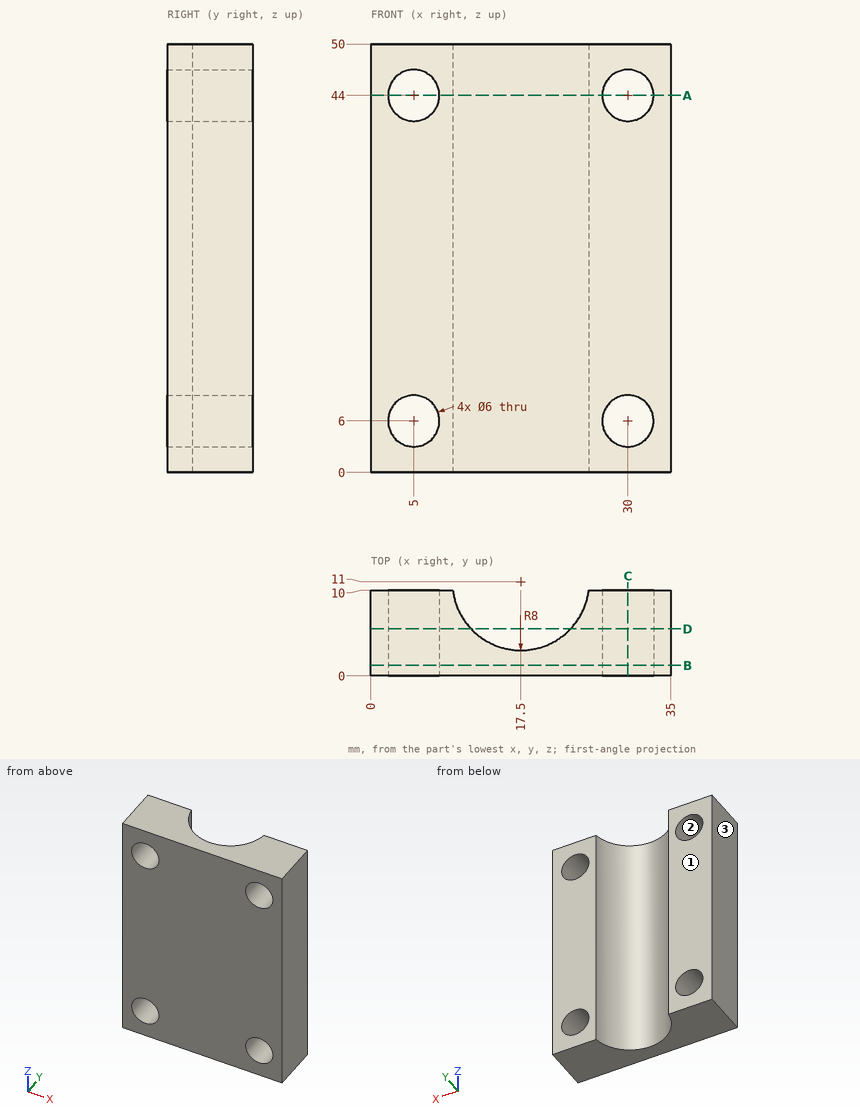
The drawing under review shows one solid part. Ordinate dimensions are in mm from its lowest x, y, z. Coordinates: 2 decimals unless noted, no trailing zeros. Order: outer loops, then holes, each group sorted by start corner. A loop starts at its lowest first (then second) coordinate and runs counter-clockwise, first axis right, second up. Notation, with made-up numbers: (-20.5, 56.5) -> (7.5, 56.5) arc R25 cw to (7.5, 93.5) -> close; hole circle Ø10 at (-37.75, 6.5). An arc over 180 degrees is marked (long way). Answer in a Markdown table with one row per item. Add a question column.
Item 1: We need section D-D on y = 5.5. Write out the cut boundary in (x, z).
Item 2: We need section C-C on x = 30. Write out the cut boundary in (y, z).
Item 3: We need section B-B on y = 1.25. Write out the cut boundary in (x, z), plus the area to 3 significant figures.
Item 4: To check wall thickness, follow probe 1 along X at (y, z) = (2.5, 44); probe 2 along Z at (x, y) = (31, 3.75); probe 3 along X at (y, z) = (8.25, 6). State the ranges of each line that lie inside material, in increasing order.
Item 5: Clearance check with a flat-ended pin moving along its axis: pin 1 (4 mm diameter, centred on x = 7, z = 21.5, fed in from -Y). State where the tip first meets the part, or that it passes through.
Item 6: Mouldability with a two-part tool opening along X and no side actions: class the marked faces 1, 2 and 3 as +X half, -X half, draft (parallel to the pull), parting line (faces both ways), or undercut.
Item 7: We need section A-A on z = 44. Write out the cut boundary in (x, y).
Final values:
| question | item | result |
|---|---|---|
| 1 | outline | (0, 0) -> (11.69, 0) -> (11.69, 50) -> (0, 50) -> close; (23.31, 0) -> (35, 0) -> (35, 50) -> (23.31, 50) -> close; hole circle Ø6 at (5, 6); hole circle Ø6 at (5, 44); hole circle Ø6 at (30, 6); hole circle Ø6 at (30, 44) |
| 2 | outline | (0, 0) -> (10, 0) -> (10, 3) -> (0, 3) -> close; (0, 9) -> (10, 9) -> (10, 41) -> (0, 41) -> close; (0, 47) -> (10, 47) -> (10, 50) -> (0, 50) -> close |
| 3 | outline | (0, 0) -> (35, 0) -> (35, 50) -> (0, 50) -> close; hole circle Ø6 at (5, 6); hole circle Ø6 at (5, 44); hole circle Ø6 at (30, 6); hole circle Ø6 at (30, 44) |
| 3 | area | 1,640 mm2 |
| 4 | probe 1 | x = 0 to 2, 8 to 27, 33 to 35 |
| 4 | probe 2 | z = 0 to 3.17, 8.83 to 41.17, 46.83 to 50 |
| 4 | probe 3 | x = 0 to 2, 8 to 9.99, 25.01 to 27, 33 to 35 |
| 5 | pin 1 | stops at y = 0 |
| 6 | face 1 | draft |
| 6 | face 2 | undercut |
| 6 | face 3 | -X half |
| 7 | outline | (0, 0) -> (2, 0) -> (2, 10) -> (0, 10) -> close; (8, 0) -> (27, 0) -> (27, 10) -> (25.44, 10) arc R8 cw to (9.56, 10) -> (8, 10) -> close; (33, 0) -> (35, 0) -> (35, 10) -> (33, 10) -> close |
